For this review, take the finished solid that the model builds, in its own axes (mm). Face numbers are marked on the shaded views. A direction names the side the tool comes from. Coordinates: 2 decimals unless noted, no trailing zeros. Order: outer loops, then holes, each group sorted by start corner. A loop starts at its lowest first (then second) coordinate and runs counter-clockwise, first axis right, second up.
from build123d import *

# Parameters (mm, degrees)
SKETCH1_R           = 25.4
BOSS_EXTRUDE2_DEPTH = 7.62
SKETCH4_R           = 4.826
CUT_EXTRUDE2_DEPTH  = 3.048
CIRPATTERN1_COUNT   = 6
SKETCH5_R           = 4.826
CUT_EXTRUDE6_DEPTH  = 3.048
SKETCH7_R           = 0.79375
CUT_EXTRUDE7_DEPTH  = 1.5875


with BuildPart() as part:
    # Sketch1 → Boss-Extrude2 (new body)
    with BuildSketch(Plane(origin=(0, 0, 0), x_dir=(1, 0, 0), z_dir=(0, 1, 0))):
        with Locations(Location((0, 0, 0), (0, 0, 270))):
            Circle(SKETCH1_R)
    extrude(amount=BOSS_EXTRUDE2_DEPTH)

    # Sketch4 → Cut-Extrude2 (cut)
    with BuildSketch(Plane(origin=(0, 0, 0), x_dir=(1, 0, 0), z_dir=(0, 1, 0))):
        with Locations(Location((0, 17.78, 0), (0, 0, 90))):
            Circle(SKETCH4_R)
    cut_extrude2 = extrude(amount=CUT_EXTRUDE2_DEPTH, mode=Mode.SUBTRACT)

    # CirPattern1: Cut-Extrude2 ×6 about axis
    cirpattern1_axis = Axis((0, 0, 0), (0, 1, 0))
    for i in range(1, CIRPATTERN1_COUNT):
        add(cut_extrude2.rotate(cirpattern1_axis, i * 360 / CIRPATTERN1_COUNT), mode=Mode.SUBTRACT)

    # Sketch5 → Cut-Extrude6 (cut)
    with BuildSketch(Plane(origin=(0, 0, 0), x_dir=(1, 0, 0), z_dir=(0, 1, 0))):
        with Locations(Location((0, 0, 0), (0, 0, 90))):
            Circle(SKETCH5_R)
    extrude(amount=CUT_EXTRUDE6_DEPTH, mode=Mode.SUBTRACT)

    # Sketch7 → Cut-Extrude7 (cut)
    with BuildSketch(Plane.XZ):
        with Locations(Location((4.532486744, 7.647788172, 0), (0, 0, 270))):
            Circle(SKETCH7_R)
        with Locations(Location((4.356935467, -7.749142748, 0), (0, 0, 270))):
            Circle(SKETCH7_R)
        with Locations(Location((-8.889422211, 0.101354577, 0), (0, 0, 270))):
            Circle(SKETCH7_R)
    extrude(amount=-CUT_EXTRUDE7_DEPTH, mode=Mode.SUBTRACT)


solid = part.part
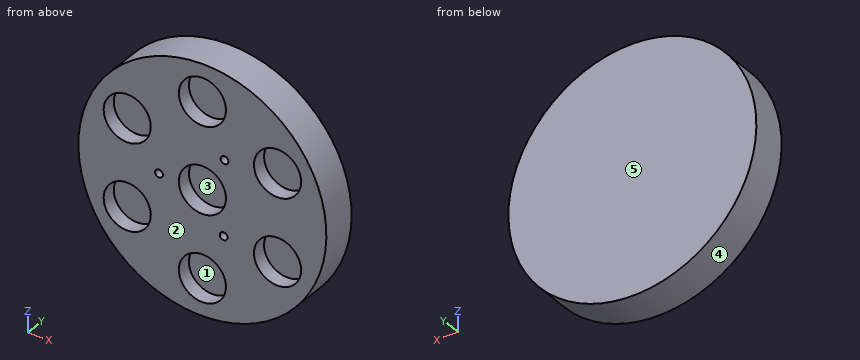
1. Take a section at C-C, the plane z = 22. Give the boundary of the cut face in (x, y).
Answer below:
outline: (-12.69, 0) - (-2.34, 0) - (-2.34, 3.05) - (2.34, 3.05) - (2.34, 0) - (12.69, 0) - (12.69, 7.62) - (-12.69, 7.62) - close
2. Take a section at B-B, the plane y = 1. Give the number of separate pieces and of enclosed holes in the cut face, plus the area to 3 significant figures.
Answer below:
separate pieces: 1
enclosed holes: 10
area: 1,510 mm2
3. Clearance check with flat-ended pins moving along their axes: pin 1 Ø5 at (x, z) = (-15.5, 8.5) entering from -Y; pin 2 Ø2 at (y, z) = (2, 9.5) entering from +X; pin 3 Ø3 at (y, z) = (4, -7.5) entering from -X. State where each tip first meets the part, or that it passes through.
Answer below:
pin 1: stops at y = 3.05
pin 2: stops at x = 23.94
pin 3: stops at x = -24.68
4. Take a section at A-A, the plane x = 0. Give the boundary of the cut face in (y, z), plus the area to 3 significant figures.
Answer below:
outline: (0, -25.4) - (7.62, -25.4) - (7.62, 25.4) - (0, 25.4) - (0, 22.61) - (3.05, 22.61) - (3.05, 12.95) - (0, 12.95) - (0, 4.83) - (3.05, 4.83) - (3.05, -4.83) - (0, -4.83) - (0, -12.95) - (3.05, -12.95) - (3.05, -22.61) - (0, -22.61) - close
area: 299 mm2
5. To check wall thickness, follow L1, parallel to Y at x = -12, z = 8; L2, parallel to X at y = 1, z = -8.89; L3, parallel to Z at x = -0.5, y = 4. State the ranges of each line that lie inside material, in increasing order.
Answer below:
L1: y = 3.05 to 7.62
L2: x = -23.79 to -20.22, -10.57 to 10.57, 20.22 to 23.79
L3: z = -25.4 to 25.4
6. The part is to be moulded in two halves that separate along X. For the marked faces 3, 4 and 5, say which applies: +X half, -X half, draft (parallel to the pull), parting line (faces both ways), or undercut.
Answer below:
face 3: undercut
face 4: parting line
face 5: draft
7. Take a section at D-D, the plane y = 3.75. Give the boundary of the cut face in (x, z), plus the area to 3 significant figures.
Answer below:
outline: circle Ø50.8 at (0, 0)
area: 2,030 mm2
8. Machinability: for the marked faces 1 and 2, which of the approach directions +Z, -Z, +X, -X, +Y, -Y give a long, thin tool a straight path to every point of the face, cutting with its end or side? Answer none if there is none.
Answer below:
face 1: -Y
face 2: +Z, -Z, +X, -X, -Y
